CAD build for the part. Positions are in the model's coordinates, mm. Give positions to 0.01 mm unless a question says otherwise; leave off trailing zeros. Loops run counter-clockwise (first coordinate to the right, second up) from the corner with the lowest first, then second, coordinate; pieces in that order, holes last.
```python
from build123d import *

# Parameters (mm, degrees)
EXTRUIR1_DEPTH = 0.1
CROQUIS2_R     = 0.5
EXTRUIR2_DEPTH = 61.742680558


with BuildPart() as part:
    # Croquis1 → Extruir1 (new body)
    with BuildSketch(Plane(origin=(0, 0, 0), x_dir=(1, 0, 0), z_dir=(0, 1, 0))):
        with BuildLine():
            Line((-33.4, 34.774386262), (-12.68172335, 34.774386262))
            ThreePointArc((-12.68172335, 34.774386262), (-10.693196053, 32.988300237), (-8.704668756, 34.774386262))
            Line((-8.704668756, 34.774386262), (11.804147498, 34.774386262))
            ThreePointArc((11.804147498, 34.774386262), (13.808796801, 34.052242285), (14.654898518, 32.096680311))
            Line((14.654898518, 32.096680311), (14.654898518, 23.480332981))
            ThreePointArc((14.654898518, 23.480332981), (14.760471327, 23.033119386), (15.054898518, 22.680332981))
            Line((15.054898518, 22.680332981), (18.254898518, 20.280332981))
            ThreePointArc((18.254898518, 20.280332981), (18.549325709, 19.927546577), (18.654898518, 19.480332981))
            Line((18.654898518, 19.480332981), (18.654898518, 8.480332981))
            ThreePointArc((18.654898518, 8.480332981), (23.890263788, -1.431262096), (35.028184679, -2.694387067))
            ThreePointArc((35.028184679, -2.694387067), (35.207188776, -2.642957473), (35.392625193, -2.625613738))
            Line((35.392625193, -2.625613738), (46.7, -2.625613738))
            ThreePointArc((46.7, -2.625613738), (47.407106781, -2.918506956), (47.7, -3.625613738))
            Line((47.7, -3.625613738), (47.7, -24.225613738))
            ThreePointArc((47.7, -24.225613738), (47.114213562, -25.6398273), (45.7, -26.225613738))
            Line((45.7, -26.225613738), (41.2, -26.225613738))
            ThreePointArc((41.2, -26.225613738), (39.361522369, -26.987136107), (38.6, -28.825613738))
            Line((38.6, -28.825613738), (38.6, -30.725613738))
            ThreePointArc((38.6, -30.725613738), (38.584277466, -33.205559421), (36.605129886, -34.7))
            Line((36.605129886, -34.7), (-25.401383808, -34.7))
            ThreePointArc((-25.401383808, -34.7), (-27.4, -32.625613738), (-29.398616192, -34.7))
            Line((-29.398616192, -34.7), (-33.4, -34.7))
            Line((-33.4, -34.7), (-33.4, -30.9))
            ThreePointArc((-33.4, -30.9), (-36, -28.3), (-38.6, -30.9))
            Line((-38.6, -30.9), (-38.6, -34.7))
            Line((-38.6, -34.7), (-47.8, -34.7))
            ThreePointArc((-47.8, -34.7), (-49.214213562, -34.114213562), (-49.8, -32.7))
            Line((-49.8, -32.7), (-49.8, -29.5))
            ThreePointArc((-49.8, -29.5), (-49.360660172, -28.439339828), (-48.3, -28))
            Line((-48.3, -28), (-45.478700604, -28))
            Line((-45.478700604, -28), (-45.478700604, -1.775613738))
            ThreePointArc((-45.478700604, -1.775613738), (-43.1, -0.125613738), (-45.478700604, 1.524386262))
            Line((-45.478700604, 1.524386262), (-45.478700604, 27.5))
            Line((-45.478700604, 27.5), (-48.3, 27.5))
            ThreePointArc((-48.3, 27.5), (-49.360660172, 27.939339828), (-49.8, 29))
            Line((-49.8, 29), (-49.8, 32.7))
            ThreePointArc((-49.8, 32.7), (-49.214213562, 34.114213562), (-47.8, 34.7))
            Line((-47.8, 34.7), (-38.6, 34.7))
            Line((-38.6, 34.7), (-38.6, 30.9))
            ThreePointArc((-38.6, 30.9), (-36, 28.3), (-33.4, 30.9))
            Line((-33.4, 30.9), (-33.4, 34.774386262))
        make_face()
    extrude(amount=EXTRUIR1_DEPTH)

    # Croquis2 → Extruir2 (cut, through all)
    with BuildSketch(Plane(origin=(0, 0.1, 0), x_dir=(1, 0, 0), z_dir=(0, 1, 0))):
        with Locations(Location((-29.478700604, 0, 0), (0, 0, 270))):
            Circle(CROQUIS2_R)
        with Locations(Location((-47.3, 32.2, 0), (0, 0, 270))):
            Circle(CROQUIS2_R)
        with Locations(Location((-47.3, -32.2, 0), (0, 0, 270))):
            Circle(CROQUIS2_R)
        with Locations(Location((12.154898518, 32.2, 0), (0, 0, 270))):
            Circle(CROQUIS2_R)
        with Locations(Location((4.521299396, 0, 0), (0, 0, 270))):
            Circle(CROQUIS2_R)
        with Locations(Location((42.7, -8.625613738, 0), (0, 0, 270))):
            Circle(CROQUIS2_R)
        with Locations(Location((42.7, -23.625613738, 0), (0, 0, 270))):
            Circle(CROQUIS2_R)
        with BuildLine():
            Line((-22.933151754, 3.5), (-21.933151754, 3.5))
            ThreePointArc((-21.933151754, 3.5), (0.521299396, 0), (-21.933151754, -3.5))
            Line((-21.933151754, -3.5), (-22.933151754, -3.5))
            Line((-22.933151754, -3.5), (-22.933151754, 3.5))
        make_face()
    extrude(amount=-EXTRUIR2_DEPTH, mode=Mode.SUBTRACT)


solid = part.part
```
1. Saw through at C-C, the plane x = -27.4. List the corners of the cut face in (y, z), and give its area (3 significant figures).
Responses:
outline: (0, -34.77) - (0.1, -34.77) - (0.1, 32.63) - (0, 32.63) - close
area: 6.74 mm2
2. Saw through at A-A, the plane x = -5.5. List the corners of the cut face in (y, z).
Responses:
outline: (0, -34.77) - (0.1, -34.77) - (0.1, -10.11) - (0, -10.11) - close; (0, 10.11) - (0.1, 10.11) - (0.1, 34.7) - (0, 34.7) - close
3. Saw through at D-D, the plane z = -16.5. List the corners of the cut face in (x, y), and give its area (3 significant figures).
Responses:
outline: (-45.48, 0) - (18.65, 0) - (18.65, 0.1) - (-45.48, 0.1) - close
area: 6.41 mm2
4. Saw through at B-B, the plane z = -7. List the corners of the cut face in (x, y), and give its area (3 significant figures).
Responses:
outline: (-45.48, 0) - (-20.1, 0) - (-20.1, 0.1) - (-45.48, 0.1) - close; (-1.85, 0) - (18.75, 0) - (18.75, 0.1) - (-1.85, 0.1) - close
area: 4.60 mm2
5. Probe line 1 along X through (y, z) = (0.05, 0); line 2 along Z through (x, y) = (-16, 0.05); line 3 along Z through (x, y) = (7, 0.05). List the from-to ranges inside material, lowest first.
Responses:
line 1: x = -43.1 to -29.98, -28.98 to -22.93, 0.52 to 4.02, 5.02 to 22.16
line 2: z = -34.77 to -10.35, 10.35 to 34.7
line 3: z = -34.77 to 34.7
6. Drop a flat-ended pin along its axis: pin 1 (18.5 mm diameter, centred on x = -10.98, z = 0, fed in from +Y). Give the stop position or say it passes through.
Responses:
pin 1: passes through
